```python
from build123d import *

# Parameters (mm, degrees)
CYLINDER002_R     = 3.5
CYLINDER002_DEPTH = 8
CYLINDER003_R     = 2
CYLINDER003_DEPTH = 25
CYLINDER001_R     = 3.5
CYLINDER001_DEPTH = 8
CYLINDER_R        = 2
CYLINDER_DEPTH    = 25
CYLINDER007_R     = 3.5
CYLINDER007_DEPTH = 8
CYLINDER006_R     = 2
CYLINDER006_DEPTH = 25
CYLINDER008_R     = 3.5
CYLINDER008_DEPTH = 8
CYLINDER009_R     = 2
CYLINDER009_DEPTH = 25
CYLINDER005_R     = 3.5
CYLINDER005_DEPTH = 8
CYLINDER004_R     = 2
CYLINDER004_DEPTH = 25
CYLINDER011_R     = 3.5
CYLINDER011_DEPTH = 8
CYLINDER010_R     = 2
CYLINDER010_DEPTH = 25
CYLINDER012_R     = 3.5
CYLINDER012_DEPTH = 8
CYLINDER013_R     = 2
CYLINDER013_DEPTH = 25
CYLINDER015_R     = 3.5
CYLINDER015_DEPTH = 8
CYLINDER014_R     = 2
CYLINDER014_DEPTH = 25
CYLINDER017_R     = 3.5
CYLINDER017_DEPTH = 8
CYLINDER016_R     = 2
CYLINDER016_DEPTH = 25
BOX_W             = 110
BOX_H             = 220
BOX_DEPTH         = 18


with BuildPart() as cilindro002:
    # Cylinder002 → Cylinder002 (new body)
    with BuildSketch(Plane(origin=(8, 17, 14), x_dir=(1, 0, 0), z_dir=(0, 0, 1))):
        Circle(CYLINDER002_R)
    extrude(amount=CYLINDER002_DEPTH)


with BuildPart() as fusion001:
    # Cylinder003 → Cylinder003 (new body)
    with BuildSketch(Plane(origin=(8, 17, 0), x_dir=(1, 0, 0), z_dir=(0, 0, 1))):
        Circle(CYLINDER003_R)
    extrude(amount=CYLINDER003_DEPTH)

    # Fusion001: union Cilindro002
    add(cilindro002.part)


with BuildPart() as fusion001_1:
    # Fusion001 placement: moved
    add(fusion001.part.moved(Location((24, 0, 0))))


with BuildPart() as cilindro001:
    # Cylinder001 → Cylinder001 (new body)
    with BuildSketch(Plane(origin=(8, 17, 14), x_dir=(1, 0, 0), z_dir=(0, 0, 1))):
        Circle(CYLINDER001_R)
    extrude(amount=CYLINDER001_DEPTH)


with BuildPart() as fusion003:
    # Cylinder → Cylinder (new body)
    with BuildSketch(Plane(origin=(8, 17, 0), x_dir=(1, 0, 0), z_dir=(0, 0, 1))):
        Circle(CYLINDER_R)
    extrude(amount=CYLINDER_DEPTH)

    # Fusion: union Cilindro001
    add(cilindro001.part)

    # Fusion003: union Fusion001
    add(fusion001_1.part)


with BuildPart() as cilindro007:
    # Cylinder007 → Cylinder007 (new body)
    with BuildSketch(Plane(origin=(8, 17, 14), x_dir=(1, 0, 0), z_dir=(0, 0, 1))):
        Circle(CYLINDER007_R)
    extrude(amount=CYLINDER007_DEPTH)


with BuildPart() as fusion006:
    # Cylinder006 → Cylinder006 (new body)
    with BuildSketch(Plane(origin=(8, 17, 0), x_dir=(1, 0, 0), z_dir=(0, 0, 1))):
        Circle(CYLINDER006_R)
    extrude(amount=CYLINDER006_DEPTH)

    # Fusion006: union Cilindro007
    add(cilindro007.part)


with BuildPart() as fusion006_1:
    # Fusion006 placement: moved
    add(fusion006.part.moved(Location((24, 0, 0))))


with BuildPart() as cilindro008:
    # Cylinder008 → Cylinder008 (new body)
    with BuildSketch(Plane(origin=(8, 17, 14), x_dir=(1, 0, 0), z_dir=(0, 0, 1))):
        Circle(CYLINDER008_R)
    extrude(amount=CYLINDER008_DEPTH)


with BuildPart() as fusion007:
    # Cylinder009 → Cylinder009 (new body)
    with BuildSketch(Plane(origin=(8, 17, 0), x_dir=(1, 0, 0), z_dir=(0, 0, 1))):
        Circle(CYLINDER009_R)
    extrude(amount=CYLINDER009_DEPTH)

    # Fusion005: union Cilindro008
    add(cilindro008.part)

    # Fusion004: union Fusion006
    add(fusion006_1.part)


with BuildPart() as fusion007_1:
    # Fusion004 placement: moved
    add(fusion007.part.moved(Location((0, 18, 0))))

    # Fusion007: union Fusion003
    add(fusion003.part)


with BuildPart() as cilindro005:
    # Cylinder005 → Cylinder005 (new body)
    with BuildSketch(Plane(origin=(8, 17, 14), x_dir=(1, 0, 0), z_dir=(0, 0, 1))):
        Circle(CYLINDER005_R)
    extrude(amount=CYLINDER005_DEPTH)


with BuildPart() as fusion002:
    # Cylinder004 → Cylinder004 (new body)
    with BuildSketch(Plane(origin=(8, 17, 0), x_dir=(1, 0, 0), z_dir=(0, 0, 1))):
        Circle(CYLINDER004_R)
    extrude(amount=CYLINDER004_DEPTH)

    # Fusion002: union Cilindro005
    add(cilindro005.part)


with BuildPart() as fusion002_1:
    # Fusion002 placement: moved
    add(fusion002.part.moved(Location((83, 83, 0))))


with BuildPart() as cilindro011:
    # Cylinder011 → Cylinder011 (new body)
    with BuildSketch(Plane(origin=(8, 17, 14), x_dir=(1, 0, 0), z_dir=(0, 0, 1))):
        Circle(CYLINDER011_R)
    extrude(amount=CYLINDER011_DEPTH)


with BuildPart() as fusion014:
    # Cylinder010 → Cylinder010 (new body)
    with BuildSketch(Plane(origin=(8, 17, 0), x_dir=(1, 0, 0), z_dir=(0, 0, 1))):
        Circle(CYLINDER010_R)
    extrude(amount=CYLINDER010_DEPTH)

    # Fusion014: union Cilindro011
    add(cilindro011.part)


with BuildPart() as fusion014_1:
    # Fusion014 placement: moved
    add(fusion014.part.moved(Location((24, 0, 0))))


with BuildPart() as cilindro012:
    # Cylinder012 → Cylinder012 (new body)
    with BuildSketch(Plane(origin=(8, 17, 14), x_dir=(1, 0, 0), z_dir=(0, 0, 1))):
        Circle(CYLINDER012_R)
    extrude(amount=CYLINDER012_DEPTH)


with BuildPart() as fusion012:
    # Cylinder013 → Cylinder013 (new body)
    with BuildSketch(Plane(origin=(8, 17, 0), x_dir=(1, 0, 0), z_dir=(0, 0, 1))):
        Circle(CYLINDER013_R)
    extrude(amount=CYLINDER013_DEPTH)

    # Fusion013: union Cilindro012
    add(cilindro012.part)

    # Fusion012: union Fusion014
    add(fusion014_1.part)


with BuildPart() as cilindro015:
    # Cylinder015 → Cylinder015 (new body)
    with BuildSketch(Plane(origin=(8, 17, 14), x_dir=(1, 0, 0), z_dir=(0, 0, 1))):
        Circle(CYLINDER015_R)
    extrude(amount=CYLINDER015_DEPTH)


with BuildPart() as fusion009:
    # Cylinder014 → Cylinder014 (new body)
    with BuildSketch(Plane(origin=(8, 17, 0), x_dir=(1, 0, 0), z_dir=(0, 0, 1))):
        Circle(CYLINDER014_R)
    extrude(amount=CYLINDER014_DEPTH)

    # Fusion009: union Cilindro015
    add(cilindro015.part)


with BuildPart() as fusion009_1:
    # Fusion009 placement: moved
    add(fusion009.part.moved(Location((24, 0, 0))))


with BuildPart() as cilindro017:
    # Cylinder017 → Cylinder017 (new body)
    with BuildSketch(Plane(origin=(8, 17, 14), x_dir=(1, 0, 0), z_dir=(0, 0, 1))):
        Circle(CYLINDER017_R)
    extrude(amount=CYLINDER017_DEPTH)


with BuildPart() as fusion015:
    # Cylinder016 → Cylinder016 (new body)
    with BuildSketch(Plane(origin=(8, 17, 0), x_dir=(1, 0, 0), z_dir=(0, 0, 1))):
        Circle(CYLINDER016_R)
    extrude(amount=CYLINDER016_DEPTH)

    # Fusion011: union Cilindro017
    add(cilindro017.part)

    # Fusion010: union Fusion009
    add(fusion009_1.part)


with BuildPart() as fusion015_1:
    # Fusion010 placement: moved
    add(fusion015.part.moved(Location((0, 18, 0))))

    # Fusion008: union Fusion012
    add(fusion012.part)


with BuildPart() as fusion015_2:
    # Fusion008 placement: moved
    add(fusion015_1.part.moved(Location((0, 83, 0))))

    # Fusion015: union Fusion007, Fusion002
    add(fusion007_1.part)
    add(fusion002_1.part)


with BuildPart() as cut:
    # Box → Box (new body)
    with BuildSketch(Plane.XY):
        with Locations((55, 110)):
            Rectangle(BOX_W, BOX_H)
    extrude(amount=BOX_DEPTH)

    # Cut: cut Fusion015
    add(fusion015_2.part, mode=Mode.SUBTRACT)


with BuildPart() as fusion016:
    # mirror: instance of Cut
    add(cut.part.mirror(Plane(origin=(110, 0, 0), x_dir=(0, -1, 0), z_dir=(1, 0, 0))))

    # Fusion016: union Cut
    add(cut.part)


solid = fusion016.part
```
Input: part model. Units: mm. Frame: model coordinates. A direction names the side the tool comes from. Coordinates: 2 decimals unless noted, no trailing zeros. Write each question's results on one line, items separated by ' | '.
Item 1: Mould query, pull axis Y, two halves, no side actions, for faces 1 (the flat face through (0, 108, 9)), 2 (the flat face through (210, 15, 14)), 3 (the flat face through (108, 220, 9)). Classes: +Y half, -Y half, draft (parallel to the pull), parting line (faces both ways), or undercut.
Conclusion:
face 1: draft | face 2: undercut | face 3: +Y half
Item 2: Pin query (flat end, axial travel): pin 1 Ø5.5 at (x, y) = (187.5, 99.5) entering from +Z. Return the tip coordinate at first contact, or that it passes through.
Conclusion:
pin 1: stops at z = 14
Item 3: Set-up query: faces 4 (the flat face through (108, 112, 0)), 5 (the flat face through (10, 33, 14)). Return all of +Z, -Z, +X, -X, +Y, -Y with unobstructed straight access to the full face (end or side cutting, diameter ignored); none if empty.
Conclusion:
face 4: -Z, +X, -X, +Y, -Y | face 5: +Z
Item 4: Material intervals for probe 1 along Y at (x, z) = (31.5, 15.5); probe 2 along Y at (x, z) = (212, 4); probe 3 along X at (y, z) = (118, 4), sorted ascending.
Conclusion:
probe 1: y = 0 to 13.54, 20.46 to 31.54, 38.46 to 96.54, 103.46 to 114.54, 121.46 to 220 | probe 2: y = 0 to 15, 19 to 33, 37 to 98, 102 to 116, 120 to 220 | probe 3: x = 0 to 6, 10 to 30, 34 to 186, 190 to 210, 214 to 220
